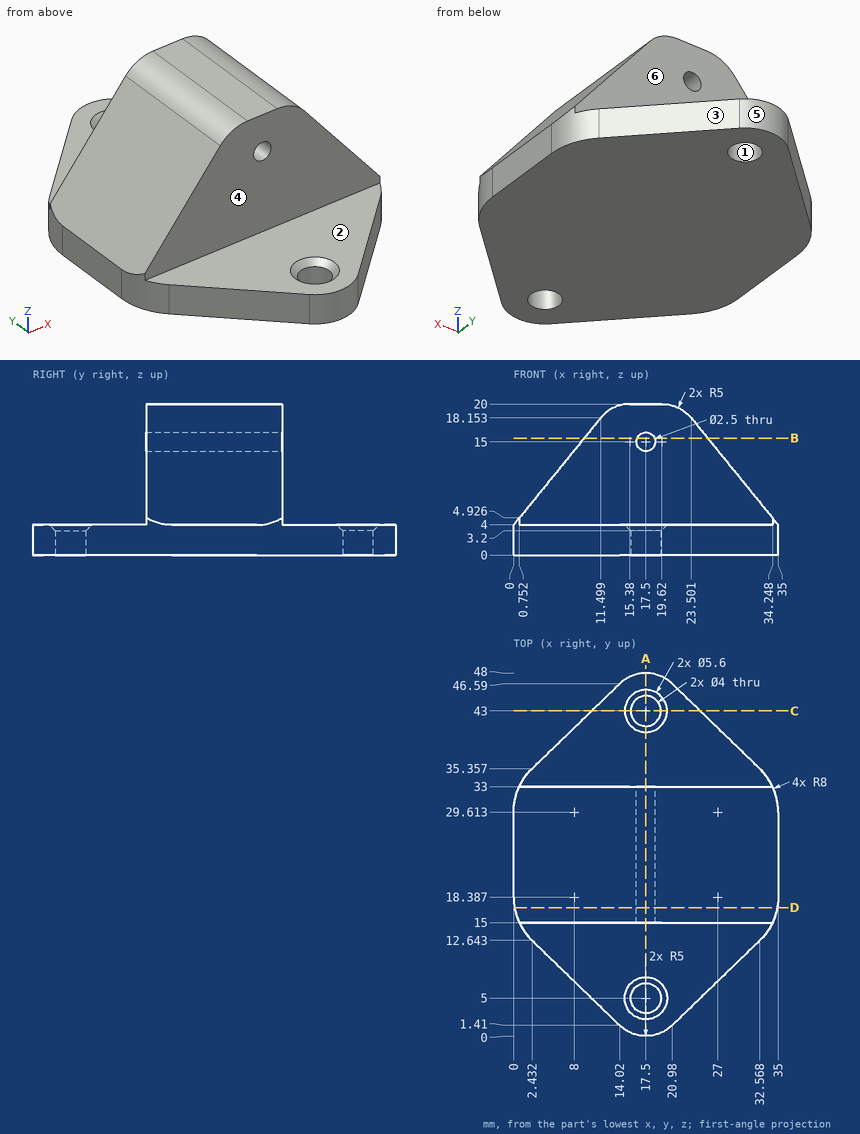
Could you check a few things on this drawing? It's one solid part, dimensions in mm from its lowest x, y, z. A direction names the side the tool comes from. Coordinates: 2 decimals unless noted, no trailing zeros. Order: outer loops, then holes, each group sorted by start corner. A loop starts at its lowest first (then second) coordinate and runs counter-clockwise, first axis right, second up. Notation, with made-up numbers: (6, -14.5) - (37, -14.5) arc R17 ccw to (37, -5.5) - close; hole circle Ø3 at (73, 20.25). An arc over 180 degrees is marked (long way). One line per question, with ' | ' between items. Start each with the question number.
1. If we mould it in two halves opening along X, with no side actions, what happens to the marked faces 1, 2 and 3? For each: released by +X, released by -X, zero draft, split by the parting line, or undercut.
2. I'm going to push flat-ended pins straight in: pin 1 Ø3 at (x, z) = (29, 4) entering from +Y; pin 2 Ø2 at (x, z) = (21, 3.5) entering from -Y; pin 3 Ø7.5 at (x, y) = (24, 37) entering from +Z; pin 4 Ø2 at (x, z) = (17.5, 15) entering from -Y. Where does each tip first touch, or does it pass through?
3. If we section it at A-A (x = 17.5): Write out the boundary of the cut face in (y, z), and give its area (3 significant figures).
4. Please list where these lines run through material, in increasing order: line 1 along Y through (x, z) = (15.5, 17.5); line 2 along Z through (x, y) = (21.5, 19); line 3 along Z through (x, y) = (17, 26) (1 decimal). Write a range as [from, to].
5. Which directions (+Z, -Z, +X, -X, +Y, -Y) give clear straight access to the entire face, cutting with the end or side of a thin tool? Please do the marked faces 4, 5 and 6.
6. If we section it at C-C (y = 43): Write out the boundary of the cut face in (x, z).
7. If we section it at B-B (z = 15.5): Write out the boundary of the cut face in (x, y) (1 decimal), and give its area (3 significant figures).
8. If we section it at D-D (y = 17): Write out the boundary of the cut face in (x, z).
Model answer:
1) face 1: undercut | face 2: zero draft | face 3: released by +X
2) pin 1: stops at y = 40.27 | pin 2: stops at y = 0.67 | pin 3: stops at z = 4 | pin 4: passes through
3) outline: (0, 0) - (3, 0) - (3, 3.2) - (2.2, 4) - (0, 4) - close; (7, 0) - (41, 0) - (41, 3.2) - (40.2, 4) - (33, 4) - (33, 13.75) - (15, 13.75) - (15, 4) - (7.8, 4) - (7, 3.2) - close; (15, 16.25) - (33, 16.25) - (33, 20) - (15, 20) - close; (45, 0) - (48, 0) - (48, 4) - (45.8, 4) - (45, 3.2) - close | area: 402 mm²
4) line 1: y = [15, 33] | line 2: z = [0, 19.63] | line 3: z = [0, 13.9], [16.1, 20]
5) face 4: +Z, +X, -X, -Y | face 5: +Z, -Z, +Y | face 6: +Z, +X, -X, +Y
6) outline: (10.32, 0) - (15.5, 0) - (15.5, 3.2) - (14.7, 4) - (10.32, 4) - close; (19.5, 0) - (24.68, 0) - (24.68, 4) - (20.3, 4) - (19.5, 3.2) - close
7) outline: (9.3, 15) - (16.4, 15) - (16.4, 33) - (9.3, 33) - close; (18.6, 15) - (25.7, 15) - (25.7, 33) - (18.6, 33) - close | area: 252 mm²
8) outline: (0.12, 0) - (34.88, 0) - (34.88, 4.15) - (23.5, 18.15) arc R5 ccw to (19.62, 20) - (15.38, 20) arc R5 ccw to (11.5, 18.15) - (0.12, 4.15) - close; hole circle Ø2.5 at (17.5, 15)
